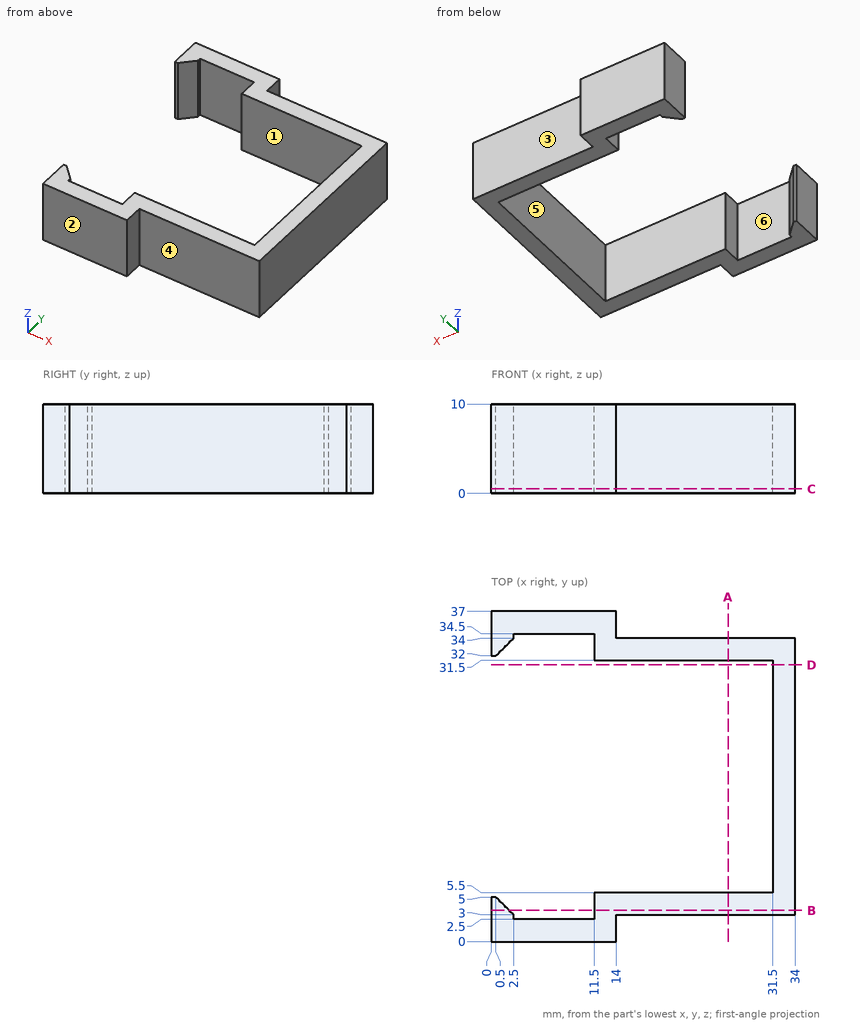
Geometry: see drawing. Coordinates: mm, zero at the bounding-box minimum. A direction names the side the tool comes from. Round coordinates to 2 decimals unless told otherwise and drop trailing zeros. Write each loop counter-clockwise with the first axis right and the second up, starting at its lowest first coordinate (ties: lowest second). Pieces come first, ordered by that corner, then holes.
1) Reachability of the marked faces 4, 5 and 6 from +Z, -Z, +X, -X, +Y, -Y: full face, straight path, thin tool, end or side. Return the list, or none.
2) Cut plane B-B (y = 3.5). Return the cut outline in (x, z), then the cut area to 3 significant figures.
3) Contact query for flat-ended pins moving along their axis: P1, Ø2, axis at x = 25, z = 1.5, coming from the +Y side; P2, Ø6, axis at x = 19, z = 3.5, coming from the -Y side; P3, Ø5, axis at y = 28, z = 6, coming from the -X side. Output: stop coordinate, or through.
4) Cut plane A-A (x = 26.5). Return the cut outline in (y, z).
5) Ray query, L1, parallel to Y at x = 23, z = 7; L2, parallel to Y at x = 11, z = 0.5; L3, parallel to X at y = 23, z = 0.75. Return the intervals inside material, ascending.
6) Draft query along Y for the marked faces 1, 2 and 3. Return one class per face: pulls with the +Y half, pulls with the -Y half, needs draft (parallel to the pull), parting line crosses it, or undercut.
7) Cut plane D-D (y = 31). Return the cut outline in (x, z).
8) Cut plane C-C (z = 0.5). Return the cut outline in (x, y).
Geometry says:
1. face 4: +Z, -Z, +X, -Y
1. face 5: +Z, -Z, -X
1. face 6: +Z, -Z
2. outline: (0, 0) - (2, 0) - (2, 10) - (0, 10) - close; (11.5, 0) - (34, 0) - (34, 10) - (11.5, 10) - close
2. area: 245 mm2
3. P1: stops at y = 34
3. P2: stops at y = 3
3. P3: stops at x = 31.5
4. outline: (3, 0) - (5.5, 0) - (5.5, 10) - (3, 10) - close; (31.5, 0) - (34, 0) - (34, 10) - (31.5, 10) - close
5. L1: y = 3 to 5.5, 31.5 to 34
5. L2: y = 0 to 2.5, 34.5 to 37
5. L3: x = 31.5 to 34
6. face 1: undercut
6. face 2: pulls with the -Y half
6. face 3: pulls with the +Y half
7. outline: (31.5, 0) - (34, 0) - (34, 10) - (31.5, 10) - close
8. outline: (0, 0) - (14, 0) - (14, 3) - (34, 3) - (34, 34) - (14, 34) - (14, 37) - (0, 37) - (0, 32) - (0.5, 32) - (2.5, 34) - (2.5, 34.5) - (11.5, 34.5) - (11.5, 31.5) - (31.5, 31.5) - (31.5, 5.5) - (11.5, 5.5) - (11.5, 2.5) - (2.5, 2.5) - (2.5, 3) - (0.5, 5) - (0, 5) - close
